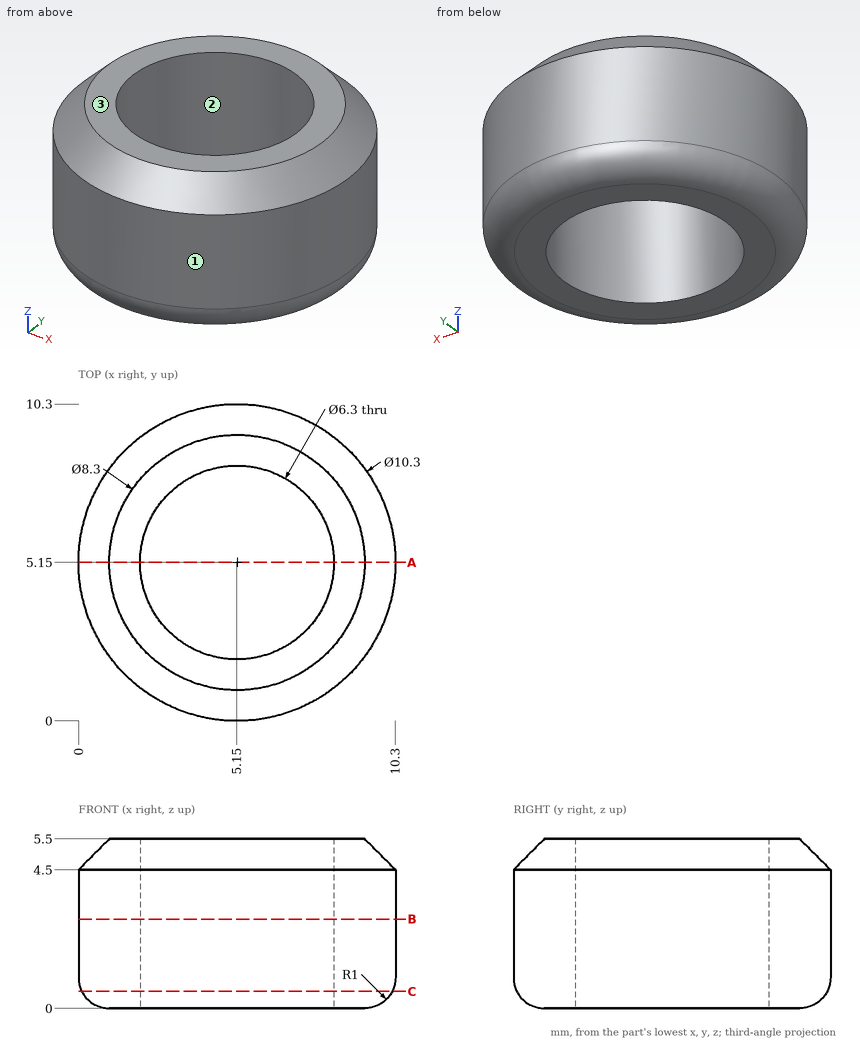
The figure shows three views and two pictorial views of one solid part (mm, origin at its lowest corner). Answer the questions. Round coordinates to 2 decimals unless told otherwise and drop trailing zeros. Write each loop counter-clockwise with the first axis right and the second up, starting at its lowest first coordinate (ties: lowest second). Pieces come first, ordered by that corner, then holes. Notation, with made-up numbers: (85, 5.5) - (141, 5.5) arc R26 ccw to (141, 20.5) - close; hole circle Ø5 at (4.5, 32). An arc over 180 degrees is marked (long way). Use one line per item in the form item = value. Start each with the question number.
Item 1: Determine the mould class of the marked faces 1, 2 and 3 for opening direction Y: +Y half, -Y half, draft (parallel to the pull), parting line (faces both ways), or undercut.
Item 2: A cutting plane is placed at B-B (z = 2.9). Write down the section's boundary in (x, y), plus the area to 3 significant figures.
Item 3: Find the intervals of material crossed by line 1 (Y direction, x = 5.15, z = 4.3); line 2 (X direction, y = 4.25, z = 0.95); line 3 (Y direction, x = 2.5, z = 1.5), in increasing order. Write a range as [from, to].
Item 4: A cutting plane is placed at C-C (z = 0.55). Write down the section's boundary in (x, y), plus the area to 3 significant figures.
Item 5: Flat-ended cylindrical pins translate along their axes: pin 1 Ø1 at (y, z) = (2, 4.5) entering from -X; pin 2 Ø1 at (y, z) = (6, 1.5) entering from +X. Find the tip coordinate at first contact, or state that the pin passes through.
Item 6: A cutting plane is placed at A-A (y = 5.15). Write down the section's boundary in (x, z).
The answers:
q1.face_1 = parting line
q1.face_2 = undercut
q1.face_3 = draft
q2.outline = circle Ø10.3 at (5.15, 5.15); hole circle Ø6.3 at (5.15, 5.15)
q2.area = 52.2 mm^2
q3.line_1 = [0, 2], [8.3, 10.3]
q3.line_2 = [0.08, 2.13], [8.17, 10.22]
q3.line_3 = [0.73, 3.45], [6.85, 9.57]
q4.outline = circle Ø10.09 at (5.15, 5.15); hole circle Ø6.3 at (5.15, 5.15)
q4.area = 48.7 mm^2
q5.pin_1 = 0.73
q5.pin_2 = 10.29
q6.outline = (0, 1) arc R1 ccw to (1, 0) - (2, 0) - (2, 5.5) - (1, 5.5) - (0, 4.5) - close; (8.3, 0) - (9.3, 0) arc R1 ccw to (10.3, 1) - (10.3, 4.5) - (9.3, 5.5) - (8.3, 5.5) - close
